Read the model definition and answer for the solid it produces. Units are mm, in the model's axes. Face numbers are marked on the shaded views. A direction names the side the tool comes from. Round coordinates to 2 decimals unless told otherwise and drop trailing zeros. Write each loop counter-clockwise with the first axis right and the second up, starting at its lowest first coordinate (ties: lowest second). Pieces come first, ordered by that corner, then holes. Notation, with made-up numbers: (24.5, -28) -> (70.5, -28) arc R11 cw to (70.5, -7) -> close; hole circle Ø11 at (75, 45.5). An arc over 180 degrees is marked (long way). Return JSON: item names as keys, results as strings. Group by question number.
(1) Straight lines are drawn through the part: line 1 (X direction, y = 3.2, z = 0) (3 decimals); line 2 (Z direction, x = 0, y = 9.5); line 3 (Y direction, x = -32.5, z = 40.5). For each, find the intervals that lie inside material, in ascending order.
(2) For the marked faces 4 and 5, determine the directions among +Z, -Z, +X, -X, +Y, -Y from which every point of the face is accessible in a straight line to the end or side of a thin tool.
(3) A cutting plane is placed at D-D on x = -32. Give the vertices of the cut face in (y, z).
(4) The mould has two halves that part along Y. Classify the marked faces 1, 2 and 3: released by +Y, released by -Y, zero draft, split by the parting line, or undercut.
(5) Given pin 1 (11 mm diameter, centred on x = -2.5, y = 0.5, fed in from +Z); pin 2 (3.5 mm diameter, centred on y = 2.5, z = -40.5, fed in from +X); pin 3 (3 mm diameter, centred on x = 33, y = -0.5, fed in from +Z); pin 4 (9 mm diameter, centred on y = -1, z = -40, fed in from -X), each flat-ended and moving along its own axis, determine where each tip first touches the part or whether it passes through.
```python
from build123d import *

# Parameters (mm, degrees)
F0_W      = 76.2
F0_H      = 88.9
F1_DEPTH  = 12.7
F4_DEPTH  = 12.7
F2_W      = 12.7
F2_H      = 12.7
F3_W      = 12.7
F3_H      = 12.7
F5_DEPTH  = 12.7
F6_R      = 1.27
F7_DEPTH  = 12.7
F8_R      = 7.9375
F9_DEPTH  = 12.7
F10_R     = 9.525
F11_DEPTH = 6.35
F12_SIZE2 = 1.26999
F12_SIZE  = 3.17499


# Not quite as in the source:
# - a fillet or chamfer is up to 0.001 mm smaller than in the source, because OpenCascade refuses the exact size


with BuildPart() as f1:
    # F0 (on Front) → F1 (new body, symmetric)
    with BuildSketch(Plane.XZ):
        Rectangle(F0_W, F0_H)
    extrude(amount=F1_DEPTH, both=True)

    # F4 (add, symmetric): faces of the model
    f4_faces = [f1.faces().sort_by_distance(p)[0] for p in [
        (-38.1, 0, 0),
        (38.1, 0, 0),
    ]]
    extrude(f4_faces, amount=F4_DEPTH, both=True, dir=(-1, 0, 0))

    # F2 (on face) + F3 (on face) → F5 (cut, symmetric)
    with BuildSketch(Plane.XY.offset(44.45)):
        with Locations((-31.75, 0)):
            Rectangle(F2_W, F2_H)
        Rectangle(F2_W, F2_H)
        with Locations((31.75, 0)):
            Rectangle(F2_W, F2_H)
    with BuildSketch(Plane(origin=(0, 0, -44.45), x_dir=(1, 0, 0), z_dir=(0, 0, -1))):
        with Locations((-31.75, 0)):
            Rectangle(F3_W, F3_H)
        Rectangle(F3_W, F3_H)
        with Locations((31.75, 0)):
            Rectangle(F3_W, F3_H)
    extrude(amount=F5_DEPTH, both=True, dir=(0, 0, 1), mode=Mode.SUBTRACT)

    # F6
    f6_edges = [f1.edges().sort_by_distance(p)[0] for p in [
        (-38.1, 0, 31.75),
        (-31.75, -6.35, 31.75),
        (-25.4, 0, 31.75),
        (-31.75, 6.35, 31.75),
        (-6.35, 0, 31.75),
        (0, -6.35, 31.75),
        (6.35, 0, 31.75),
        (0, 6.35, 31.75),
        (31.75, -6.35, 31.75),
        (38.1, 0, 31.75),
        (31.75, 6.35, 31.75),
        (25.4, 0, 31.75),
        (-31.75, 6.35, -31.75),
        (-25.4, 0, -31.75),
        (-31.75, -6.35, -31.75),
        (-38.1, 0, -31.75),
        (6.35, 0, -31.75),
        (0, -6.35, -31.75),
        (-6.35, 0, -31.75),
        (0, 6.35, -31.75),
        (31.75, 6.35, -31.75),
        (38.1, 0, -31.75),
        (31.75, -6.35, -31.75),
        (25.4, 0, -31.75),
    ]]
    fillet(f6_edges, radius=F6_R)

    # F7 (cut, symmetric): faces of the model
    f7_faces = [f1.faces().sort_by_distance(p)[0] for p in [
        (50.8, 0, 0),
        (-50.8, 0, 0),
    ]]
    extrude(f7_faces, amount=F7_DEPTH, both=True, dir=(1, 0, 0), mode=Mode.SUBTRACT)

    # F8 (on face) → F9 (cut)
    with BuildSketch(Plane(origin=(0, 12.7, 0), x_dir=(-1, 0, 0), z_dir=(0, 1, 0))):
        Circle(F8_R)
    extrude(amount=-F9_DEPTH, mode=Mode.SUBTRACT)

    # F10 (on face) → F11 (cut)
    with BuildSketch(Plane(origin=(0, 0, 0), x_dir=(-1, 0, 0), z_dir=(0, 1, 0))):
        Circle(F10_R)
    extrude(amount=F11_DEPTH, mode=Mode.SUBTRACT)

    # F12 (size 3.175 and 1.27 in the source; OpenCascade refuses exactly that, so slightly less here)
    f12_edges = [f1.edges().sort_by_distance(p)[0] for p in [
        (9.525, 0, 0),
        (9.525, 6.35, 0),
    ]]
    f12_side = f1.faces().sort_by_distance((9.525, 3.175, 0))[0]
    chamfer(f12_edges, length=F12_SIZE, length2=F12_SIZE2, reference=f12_side)


solid = f1.part
```
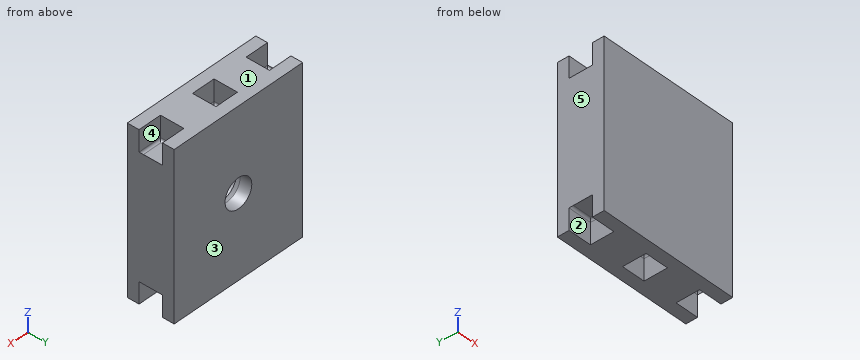
Checks:
{
 "1": {"line 1": "x = -38.1 to -9.515, 9.515 to 38.1", "line 2": "z = -44.45 to -7.94, 7.94 to 44.45", "line 3": "y = -12.7 to -6.35, 6.35 to 12.7"},
 "2": {"face 4": "+Z, +X", "face 5": "+Z, -Z, -X, +Y, -Y"},
 "3": {"outline": "(-12.7, -44.45) -> (-6.35, -44.45) -> (-6.35, -33.02) arc R1.27 cw to (-5.08, -31.75) -> (5.08, -31.75) arc R1.27 cw to (6.35, -33.02) -> (6.35, -44.45) -> (12.7, -44.45) -> (12.7, 44.45) -> (6.35, 44.45) -> (6.35, 33.02) arc R1.27 cw to (5.08, 31.75) -> (-5.08, 31.75) arc R1.27 cw to (-6.35, 33.02) -> (-6.35, 44.45) -> (-12.7, 44.45) -> close"},
 "4": {"face 1": "zero draft", "face 2": "undercut", "face 3": "released by +Y"},
 "5": {"pin 1": "stops at z = 44.45", "pin 2": "stops at x = 25.4", "pin 3": "stops at z = 31.75", "pin 4": "stops at x = -25.4"}
}
